Model file for the job. Use its own axes, mm. Face numbers are marked on the shaded views. Coordinates: 2 decimals unless noted, no trailing zeros. Order: outer loops, then holes, each group sorted by start corner. A loop starts at its lowest first (then second) coordinate and runs counter-clockwise, first axis right, second up. Notation, with made-up numbers: (-11, 61.25) - (-5, 61.25) arc R9 ccw to (-5, 77.25) - close; hole circle Ø5 at (73, 43). An arc over 180 degrees is marked (long way). Put each result on its own line as item: value. Start each with the question number.
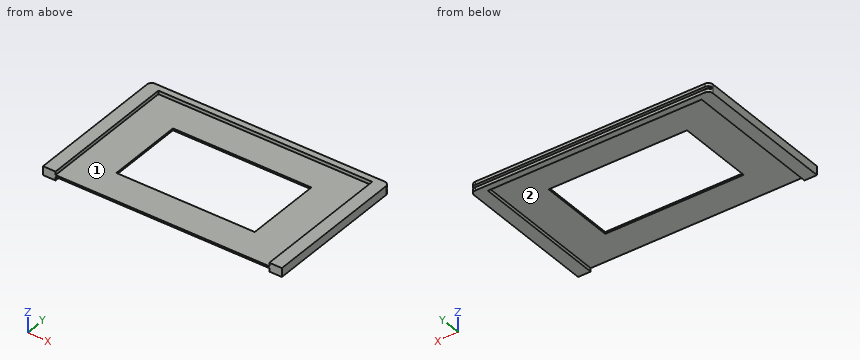
```python
from build123d import *

# Parameters (mm, degrees)
EXTRUDE_1_DEPTH     = 7
CUT_EXTRUDE_1_DEPTH = 2.75
CUT_EXTRUDE_2_DEPTH = 2.75
SKETCH_4_W          = 190.2
SKETCH_4_H          = 2
CUT_EXTRUDE_3_DEPTH = 2.5
SKETCH_5_W          = 110.2
SKETCH_5_H          = 61.2
CUT_EXTRUDE_4_DEPTH = 118.847914448


with BuildPart() as part:
    # 草图1 → 凸台-拉伸1 (new body)
    with BuildSketch(Plane.XY):
        with BuildLine():
            Line((-91.35, 69.469838346), (91.35, 69.469838346))
            ThreePointArc((91.35, 69.469838346), (94.001650429, 68.371488775), (95.1, 65.719838346))
            Line((95.1, 65.719838346), (95.1, -46.730161654))
            Line((95.1, -46.730161654), (-95.1, -46.730161654))
            Line((-95.1, -46.730161654), (-95.1, 65.719838346))
            ThreePointArc((-95.1, 65.719838346), (-94.001650429, 68.371488775), (-91.35, 69.469838346))
        make_face()
    extrude(amount=EXTRUDE_1_DEPTH)

    # 草图2 → 切除-拉伸1 (cut)
    with BuildSketch(Plane.XY):
        Polygon((-85.1, -46.730161654), (85.1, -46.730161654), (85.1, -36.730161654), (85.1, 59.469838346), (85.1, 64.469838346), (-85.1, 64.469838346), (-85.1, 59.469838346), (-85.1, -36.730161654), align=None)
    extrude(amount=CUT_EXTRUDE_1_DEPTH, mode=Mode.SUBTRACT)

    # 草图3 → 切除-拉伸2 (cut)
    with BuildSketch(Plane.XY.offset(7)):
        Polygon((-85.1, -36.730161654), (-85.1, -46.730161654), (85.1, -46.730161654), (85.1, -36.730161654), (85.1, 59.469838346), (85.1, 64.469838346), (-85.1, 64.469838346), (-85.1, 59.469838346), align=None)
    extrude(amount=-CUT_EXTRUDE_2_DEPTH, mode=Mode.SUBTRACT)

    # 草图4 → 切除-拉伸3 (cut)
    with BuildSketch(Plane(origin=(0, 69.469838346, 0), x_dir=(1, 0, 0), z_dir=(0, 1, 0))):
        with Locations((0, -3.5)):
            Rectangle(SKETCH_4_W, SKETCH_4_H)
    extrude(amount=-CUT_EXTRUDE_3_DEPTH, mode=Mode.SUBTRACT)

    # 草图5 → 切除-拉伸4 (cut, through all)
    with BuildSketch(Plane.XY.offset(4.25)):
        with Locations((0, 8.869838346)):
            Rectangle(SKETCH_5_W, SKETCH_5_H)
    extrude(amount=-CUT_EXTRUDE_4_DEPTH, mode=Mode.SUBTRACT)


solid = part.part
```
Item 1: Slice it at B-B, the plane y = -1. Give the cut face in (x, z).
Item 2: Wall check: line 1 along X through (y, z) = (-14, 4.75); line 2 along X through (y, z) = (-20.5, 3); line 3 along Y through (x, z) = (46.5, 3.75). Give the ranges that are in metal, low to high.
Item 3: Pull direction X, two halves, no side cores. Call the marked faces 1 and 2: pulls with the +X half, pulls with the -X half, needs draft (parallel to the pull), parting line crosses it, or undercut.
Item 4: Slice it at A-A, the plane x = 49. Give the cut face in (y, z), plus the area to 3 significant figures.
Item 5: Slice it at C-C, the plane y = -26.5. Give the cut face in (x, z), plus the area to 3 significant figures.
Item 6: Flat gauge pins, fed straight in: pin 1 Ø1 at (x, y) = (-16.5, 57) entering from +Z; pin 2 Ø4 at (x, y) = (-67.5, 14) entering from -Z; pin 3 Ø0.8 at (x, z) = (-6, 4) entering from +Y. Where does each tip first touch, or does it go through?
Item 7: Slice it at D-D, the plane x = -58. Give the cut face in (y, z).
Here are the results:
1. outline: (-95.1, 0) - (-85.1, 0) - (-85.1, 2.75) - (-55.1, 2.75) - (-55.1, 4.25) - (-85.1, 4.25) - (-85.1, 7) - (-95.1, 7) - close; (55.1, 2.75) - (85.1, 2.75) - (85.1, 0) - (95.1, 0) - (95.1, 7) - (85.1, 7) - (85.1, 4.25) - (55.1, 4.25) - close
2. line 1: x = -95.1 to -85.1, 85.1 to 95.1
2. line 2: x = -95.1 to -55.1, 55.1 to 95.1
2. line 3: y = -46.73 to -21.73, 39.47 to 66.97
3. face 1: undercut
3. face 2: undercut
4. outline: (-46.73, 2.75) - (-21.73, 2.75) - (-21.73, 4.25) - (-46.73, 4.25) - close; (39.47, 2.75) - (64.47, 2.75) - (64.47, 0) - (69.47, 0) - (69.47, 2.5) - (66.97, 2.5) - (66.97, 4.5) - (69.47, 4.5) - (69.47, 7) - (64.47, 7) - (64.47, 4.25) - (39.47, 4.25) - close
4. area: 105 mm^2
5. outline: (-95.1, 0) - (-85.1, 0) - (-85.1, 2.75) - (85.1, 2.75) - (85.1, 0) - (95.1, 0) - (95.1, 7) - (85.1, 7) - (85.1, 4.25) - (-85.1, 4.25) - (-85.1, 7) - (-95.1, 7) - close
5. area: 395 mm^2
6. pin 1: stops at z = 4.25
6. pin 2: stops at z = 2.75
6. pin 3: stops at y = 66.97
7. outline: (-46.73, 2.75) - (64.47, 2.75) - (64.47, 0) - (69.47, 0) - (69.47, 2.5) - (66.97, 2.5) - (66.97, 4.5) - (69.47, 4.5) - (69.47, 7) - (64.47, 7) - (64.47, 4.25) - (-46.73, 4.25) - close
